Check sheet for the modelled part. Datum: model origin and axes. Units: mm. A direction names the side the tool comes from. Round coordinates to 2 decimals unless told otherwise and drop trailing zeros. Loops run counter-clockwise (first coordinate to the right, second up) from the corner with the lowest first, then second, coordinate; pieces in that order, holes last. Notation, with made-up numbers: (76, 4) - (85, 4) arc R28 cw to (85, 22) - close; hole circle Ø2 at (-40, 26.5). An arc over 180 degrees is marked (long way). Answer in a Markdown table with one row per item. Add a question column.
(1) Mould release check, pull along Z, two halves, no side actions. Record for faces 3 (the flat face through (49, -5, 0)), 4 (the flat face through (0, -5, 45)), 5 (the cylindrical face through (410.432, -5.07, 39.638)), 6 (the flat face through (276, -5, 90.7)): +Z half, -Z half, draft (parallel to the pull), parting line (faces both ways), or undercut.
(2) Thickness scan on line 1 along Z through (x, y) = (442.5, -4.25); line 2 along X through (y, z) = (-7.25, 52); line 3 along Z through (x, y) = (397.5, -7.25). Record the ranges inside material, lowest first.
(3) Cross-section at B-B on y = -3.25. Enter the section's corners in (x, z), then the cut area to 3 significant figures.
(4) Cross-section at A-A on x = 280. Enter the section's corners in (y, z), then the cut area to 3 significant figures.
(5) Gauge pin test, flat ends, axial feed: pin 1 (22.5 mm diameter, centred on x = 280, z = 35, fed in from -Y); pin 2 (8 mm diameter, centred on x = 473.5, z = 79, fed in from +Y); pin 3 (3 mm diameter, centred on x = 132, y = -7.5, fed in from -Z). Record the tip position at first contact, or that the pin passes through.
(6) Access from +Z, -Z, +X, -X, +Y, -Y to the whole of each face (thin tool, end or side, straight path). Record for faces 1 (the flat face through (276, -10, 56)), 2 (the flat face through (460, -5, 5)).
from build123d import *

# Parameters (mm, degrees)
SKETCH_W        = 560
SKETCH_H        = 90.7
PAD_DEPTH       = 10
SKETCH001_R     = 14
POCKET_DEPTH    = 10.001
SKETCH002_W     = 50
SKETCH002_H     = 10
POCKET001_DEPTH = 10.001


with BuildPart() as part:
    # Sketch → Pad (new body)
    with BuildSketch(Plane.XZ):
        with Locations((280, 45.35)):
            Rectangle(SKETCH_W, SKETCH_H)
    extrude(amount=PAD_DEPTH)

    # Sketch001 → Pocket (cut, through all)
    with BuildSketch(Plane.XZ.offset(10)):
        with Locations((117.5, 45)):
            Circle(SKETCH001_R)
        with Locations((162.5, 45)):
            Circle(SKETCH001_R)
        with Locations((397.5, 45)):
            Circle(SKETCH001_R)
        with Locations((442.5, 45)):
            Circle(SKETCH001_R)
        with Locations((280, 35)):
            Circle(SKETCH001_R)
    extrude(amount=-POCKET_DEPTH, mode=Mode.SUBTRACT)

    # Sketch002 → Pocket001 (cut, through all)
    with BuildSketch(Plane.XZ.offset(10)):
        with Locations((125, 5)):
            Rectangle(SKETCH002_W, SKETCH002_H)
        with Locations((435, 5)):
            Rectangle(SKETCH002_W, SKETCH002_H)
    extrude(amount=-POCKET001_DEPTH, mode=Mode.SUBTRACT)


solid = part.part
Answers:
| question | item | result |
|---|---|---|
| 1 | face 3 | -Z half |
| 1 | face 4 | draft |
| 1 | face 5 | undercut |
| 1 | face 6 | +Z half |
| 2 | line 1 | z = 10 to 31, 59 to 90.7 |
| 2 | line 2 | x = 0 to 105.38, 129.62 to 150.38, 174.62 to 385.38, 409.62 to 430.38, 454.62 to 560 |
| 2 | line 3 | z = 0 to 31, 59 to 90.7 |
| 3 | outline | (0, 0) - (100, 0) - (100, 10) - (150, 10) - (150, 0) - (410, 0) - (410, 10) - (460, 10) - (460, 0) - (560, 0) - (560, 90.7) - (0, 90.7) - close; hole circle Ø28 at (117.5, 45); hole circle Ø28 at (162.5, 45); hole circle Ø28 at (280, 35); hole circle Ø28 at (397.5, 45); hole circle Ø28 at (442.5, 45) |
| 3 | area | 46,700 mm^2 |
| 4 | outline | (-10, 0) - (0, 0) - (0, 21) - (-10, 21) - close; (-10, 49) - (0, 49) - (0, 90.7) - (-10, 90.7) - close |
| 4 | area | 627 mm^2 |
| 5 | pin 1 | passes through |
| 5 | pin 2 | stops at y = 0 |
| 5 | pin 3 | stops at z = 10 |
| 6 | face 1 | +Z, -Z, +X, -X, -Y |
| 6 | face 2 | -Z, +Y, -Y |
